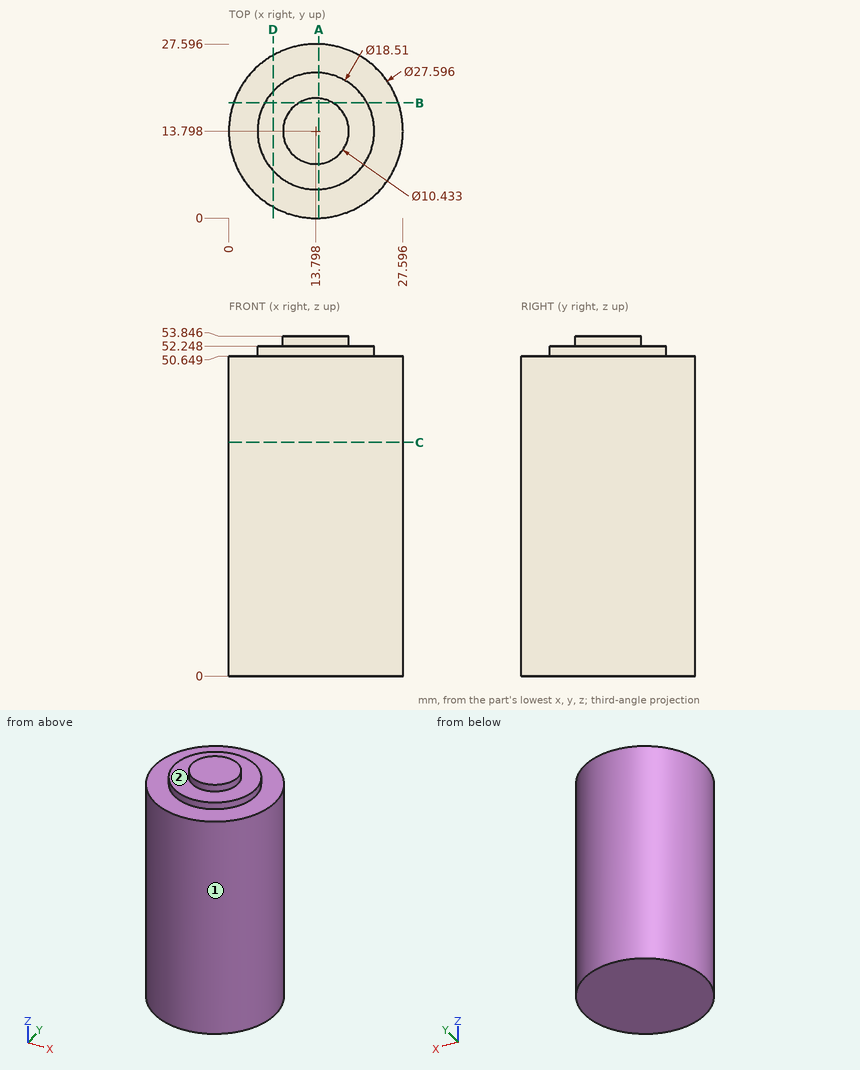
Here's the drawing with two shaded views (mm, measured from the low corner). I have some questions. A direction names the side the tool comes from. Round coordinates to 2 decimals unless told otherwise and drop trailing zeros. Write each loop counter-clockwise with the first axis right and the second up, starting at its lowest first coordinate (ties: lowest second). Pieces come first, ordered by that corner, then holes.
(1) If I drill on probe 1 along Z at (x, y) = (7.5, 12.75); probe 2 along Z at (x, y) = (15.5, 1.75); probe 3 along Y at (x, z) = (9, 43.5) (1 decimal), over which ranges is the centre line in solid material (lowest first)?
Findings below:
probe 1: z = 0 to 52.25
probe 2: z = 0 to 50.65
probe 3: y = 0.9 to 26.7
(2) For pin 1 (5 mm diameter, centred on x = 3, z = 27.5, fed in from +Y); pin 2 (2 mm diameter, centred on x = 17, y = 4.5, fed in from +Z); pin 3 (2 mm diameter, centred on y = 19, z = 40, fed in from -X) (1 decimal), each with a flat end and sliding along its axis, tell me the tip position at first contact or that it passes through.
Findings below:
pin 1: stops at y = 24.82
pin 2: stops at z = 52.25
pin 3: stops at x = 0.7
(3) Suppose I cut it at B-B on y = 18.25. Write out the boundary of the cut face in (x, z) (1 decimal).
Findings below:
outline: (0.7, 0) - (26.9, 0) - (26.9, 50.6) - (21.9, 50.6) - (21.9, 52.2) - (16.5, 52.2) - (16.5, 53.8) - (11.1, 53.8) - (11.1, 52.2) - (5.7, 52.2) - (5.7, 50.6) - (0.7, 50.6) - close
(4) Suppose I cut it at D-D on x = 7. Write out the boundary of the cut face in (y, z) (1 decimal).
Findings below:
outline: (1.8, 0) - (25.8, 0) - (25.8, 50.6) - (20.1, 50.6) - (20.1, 52.2) - (7.5, 52.2) - (7.5, 50.6) - (1.8, 50.6) - close
(5) Which directions (+Z, -Z, +X, -X, +Y, -Y) give clear straight access to the entire face, cutting with the end or side of a thin tool? Please do the marked faces 1 and 2.
Findings below:
face 1: +Z, -Z
face 2: +Z
(6) Suppose I cut it at A-A on x = 14.25. Write out the boundary of the cut face in (y, z) (1 decimal), and give its area (3 significant figures).
Findings below:
outline: (0, 0) - (27.6, 0) - (27.6, 50.6) - (23, 50.6) - (23, 52.2) - (19, 52.2) - (19, 53.8) - (8.6, 53.8) - (8.6, 52.2) - (4.6, 52.2) - (4.6, 50.6) - (0, 50.6) - close
area: 1,440 mm2
(7) Suppose I cut it at C-C on z = 37. Write out the boundary of the cut face in (x, y), and give its area (3 significant figures).
Findings below:
outline: circle Ø27.6 at (13.8, 13.8)
area: 598 mm2
